```python
from build123d import *


with BuildPart() as part:
    # Sketch1 → Revolve1 (revolve)
    with BuildSketch(Plane(origin=(0, 0, 0), x_dir=(1, 0, 0), z_dir=(0, 1, 0)), mode=Mode.PRIVATE) as revolve1_sk:
        with BuildLine():
            Line((-3.5, 10), (-3.5, 9.5))
            ThreePointArc((-3.5, 9.5), (-1, 7), (1.5, 9.5))
            Line((1.5, 9.5), (1.5, 10))
            Line((1.5, 10), (3.25, 10))
            Line((3.25, 10), (3.25, 9.5))
            ThreePointArc((3.25, 9.5), (5.75, 7), (8.25, 9.5))
            Line((8.25, 9.5), (8.25, 10))
            Line((8.25, 10), (10, 10))
            Line((10, 10), (10, 4))
            Line((10, 4), (-10, 4))
            Line((-10, 4), (-10, 10))
            Line((-10, 10), (-3.5, 10))
        make_face()
    revolve(revolve1_sk.sketch.rotate(Axis((-17.222797871, 0, 0), (1, 0, 0)), 180), axis=Axis((-17.222797871, 0, 0), (1, 0, 0)))


solid = part.part
```
CAD build for the part. Positions are in the model's coordinates, mm. A direction names the side the tool comes from. Coordinates: 2 decimals unless noted, no trailing zeros. Loops run counter-clockwise (first coordinate to the right, second up) from the corner with the lowest first, then second, coordinate; pieces in that order, holes last. Notation, with made-up numbers: (31.5, 29) - (69.5, 29) arc R20 ccw to (69.5, 61) - close; hole circle Ø1 at (54, -34). An arc over 180 degrees is marked (long way). Return JSON: item names as keys, results as strings.
1. Band-saw the part on D-D (x = 4). Give the cut face in (y, z).
Result:
{"outline": "circle Ø15.43 at (0, 0); hole circle Ø8 at (0, 0)"}
2. 3-axis set-ups, long thin cutter, end or side, ignore diameter. For faces 4 (the flat face through (8.25, 4, -9)), 5 (the cylindrical face through (-7, 0, -10)): which of +Z, -Z, +X, -X, +Y, -Y reach the whole face in a straight line?
Result:
{"face 4": "none", "face 5": "+X, -X"}
3. Band-saw the part on C-C (y = -8.5). State how many separate pieces and enclosed holes the cut face has, and give its area (3 significant figures).
Result:
{"separate pieces": "3", "enclosed holes": "0", "area": "109 mm2"}
4. Probe L1, parallel to X at y = -3.5, z = 9; L2, parallel to X at y = 4, z = -7.5; L3, parallel to Y at x = 2.5, z = 0. List the from-to ranges inside material, lowest first. Write a range as from..to.
Result:
{"L1": "x = -10..-3.5, 1.5..3.25, 8.25..10", "L2": "x = -10..-3.29, 1.29..3.46, 8.04..10", "L3": "y = -10..-4, 4..10"}
5. Mould opens along X. For faces 1 (the cylindrical face through (9, 0, -10)), 2 (the flat face through (10, -0.1, 4.3)), 3 (the flat face through (-3.5, 4, 9)) say: released by +X, released by -X, zero draft, split by the parting line, or undercut.
Result:
{"face 1": "zero draft", "face 2": "released by +X", "face 3": "undercut"}
6. Drop flat-ended pins along their axis: pin 1 (4 mm diameter, centred on x = 7.5, z = 3.5, fed in from -Y); pin 2 (3 mm diameter, centred on x = 1, z = 4, fed in from -Y); pin 3 (1.5 mm diameter, centred on x = -5, y = -7, fed in from +Z); pin 4 (1.5 mm diameter, centred on y = -2, z = 2.5, fed in from +X). Give the stop position or say it passes through.
Result:
{"pin 1": "stops at y = -9.86", "pin 2": "stops at y = -9.66", "pin 3": "stops at z = 7.81", "pin 4": "passes through"}
7. Band-saw the part on A-A (z = 0). Give the cut face in (x, y), and give its area (3 significant figures).
Result:
{"outline": "(-10, -10) - (-3.5, -10) - (-3.5, -9.5) arc R2.5 cw to (1.5, -9.5) - (1.5, -10) - (3.25, -10) - (3.25, -9.5) arc R2.5 cw to (8.25, -9.5) - (8.25, -10) - (10, -10) - (10, -4) - (-10, -4) - close; (-10, 4) - (10, 4) - (10, 10) - (8.25, 10) - (8.25, 9.5) arc R2.5 cw to (3.25, 9.5) - (3.25, 10) - (1.5, 10) - (1.5, 9.5) arc R2.5 cw to (-3.5, 9.5) - (-3.5, 10) - (-10, 10) - close", "area": "191 mm2"}
